Here's how the part is built. I have some questions about the finished solid (model axes, mm). Round coordinates to 2 decimals unless told otherwise and drop trailing zeros. Order: outer loops, then holes, each group sorted by start corner. A loop starts at its lowest first (then second) coordinate and runs counter-clockwise, first axis right, second up. Notation, with made-up numbers: (-18, -26) -> (15, -26) arc R7 cw to (15, -22) -> close; hole circle Ø8 at (87, 76). An arc over 180 degrees is marked (long way). Use a Markdown table: item, result. Add a question column.
(1) I'm going to push flat-ended pins straight in: P1, Ø3.5, axis at x = -5, z = 8, coming from the +Y side; P2, Ø10, axis at y = 72, z = 5, coming from the +X side; P3, Ø5, axis at x = -40.5, y = -55.5, coming from the +Z side; P4, Ø4.5, axis at y = -86.36, z = 11.11, coming from the -X side. Where does each tip first touch, or does it pass through?
(2) I want a section at B-B, the plane x = 0. Please give me the cut outline in (y, z).
(3) I want a section at A-A, the plane y = 86.36. Give the number of separate pieces and of enclosed holes in the cut face, then the cut area to 3 significant figures.
(4) I want a section at D-D, the plane x = 69. Please give me the cut outline in (y, z).
(5) If I drill on probe 1 along Z at (x, y) = (5.1, 86.36); probe 2 along Z at (x, y) = (-1, -31.5); probe 3 along Z at (x, y) = (4, -86), over which ranges is the centre line in solid material (lowest first)?
from build123d import *

# Parameters (mm, degrees)
F0_W     = 203.2
F0_H     = 203.2
F1_DEPTH = 4.7625
F2_W     = 17.78
F2_H     = 12.7
F3_DEPTH = 6.35
F4_W     = 6.35
F4_H     = 17.78
F4_W_2   = 3.175
F5_DEPTH = 12.7
F7_D     = 4.7625
F9_DEPTH = 4.7635
F10_R    = 6.35
F12_D    = 2.794


with BuildPart() as f1:
    # F0 (on Top) → F1 (new body)
    with BuildSketch(Plane.XY):
        Rectangle(F0_W, F0_H)
    extrude(amount=F1_DEPTH)

    # F2 (on Right) → F3 (join, symmetric)
    with BuildSketch(Plane.YZ):
        with Locations((-86.36, 11.1125)):
            Rectangle(F2_W, F2_H)
        with Locations((86.36, 11.1125)):
            Rectangle(F2_W, F2_H)
    extrude(amount=F3_DEPTH, both=True)

    # F4 (on face) → F5 (cut, through all)
    with BuildSketch(Plane.XY.offset(17.4625)):
        with Locations((0, -86.36)):
            Rectangle(F4_W, F4_H)
        with Locations((-1.5875, 86.36)):
            Rectangle(F4_W_2, F4_H)
        with Locations((1.5875, 86.36)):
            Rectangle(F4_W_2, F4_H)
    extrude(amount=-F5_DEPTH, mode=Mode.SUBTRACT)

    # F7 (through all)
    with Locations(Plane.YZ.offset(6.35)):
        with Locations((-86.36, 11.1125), (86.36, 11.1125)):
            Hole(F7_D / 2)

    # F8 (on face) → F9 (cut, through all)
    with BuildSketch(Plane.XY.offset(4.7625)):
        with BuildLine():
            Line((-101.6, -101.6), (-3.53e-08, -101.6))
            ThreePointArc((-3.53e-08, -101.6), (-71.842048981, -71.8420489561), (-101.6, 0))
            Line((-101.6, 0), (-101.6, -101.6))
        make_face()
        with BuildLine():
            ThreePointArc((-101.6, 0), (-71.8420489199, 71.8420490172), (1.376e-07, 101.6))
            Line((1.376e-07, 101.6), (-101.6, 101.6))
            Line((-101.6, 101.6), (-101.6, 0))
        make_face()
        with BuildLine():
            ThreePointArc((1.376e-07, 101.6), (71.8420490172, 71.8420489199), (101.6, 0))
            Line((101.6, 0), (101.6, 101.6))
            Line((101.6, 101.6), (1.376e-07, 101.6))
        make_face()
        with BuildLine():
            Line((101.6, -101.6), (101.6, 0))
            ThreePointArc((101.6, 0), (71.8420489561, -71.842048981), (-3.53e-08, -101.6))
            Line((-3.53e-08, -101.6), (101.6, -101.6))
        make_face()
    extrude(amount=-F9_DEPTH, mode=Mode.SUBTRACT)

    # F10
    f10_edges = [f1.edges().sort_by_distance(p)[0] for p in [
        (-4.7625, -95.25, 17.4625),
        (-4.7625, -77.47, 17.4625),
        (-4.7625, 77.47, 17.4625),
        (-4.7625, 95.25, 17.4625),
        (4.7625, 95.25, 17.4625),
        (4.7625, 77.47, 17.4625),
        (4.7625, -95.25, 17.4625),
        (4.7625, -77.47, 17.4625),
    ]]
    fillet(f10_edges, radius=F10_R)

    # F12 (through all)
    with Locations(Plane.XY.offset(4.7625)):
        with Locations((-88.9, 0), (88.9, 0), (-96.52, 0), (96.52, 0)):
            Hole(F12_D / 2)


solid = f1.part
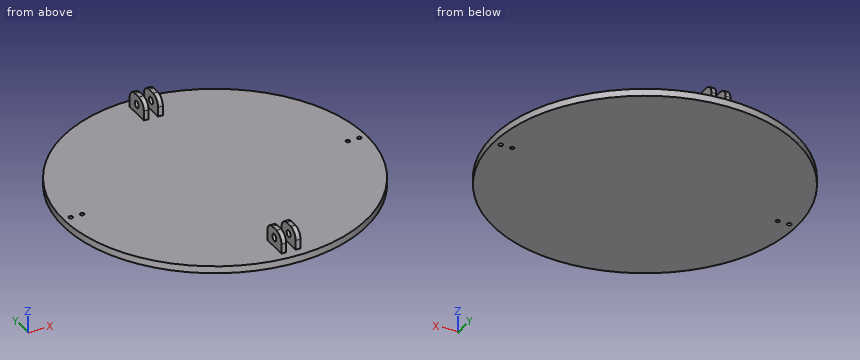
Taken from the geometry:
| question | item | result |
|---|---|---|
| 1 | P1 | stops at y = 95.25 |
| 1 | P2 | stops at x = 76.37 |
| 1 | P3 | stops at z = 4.76 |
| 1 | P4 | passes through |
| 2 | outline | (-101.6, 0) -> (101.6, 0) -> (101.6, 4.76) -> (-101.6, 4.76) -> close |
| 3 | separate pieces | 3 |
| 3 | enclosed holes | 0 |
| 3 | area | 560 mm2 |
| 4 | outline | (-74.58, 0) -> (74.58, 0) -> (74.58, 4.76) -> (-74.58, 4.76) -> close |
| 5 | probe 1 | z = 0 to 8.73, 13.49 to 17.46 |
| 5 | probe 2 | z = 0 to 4.76 |
| 5 | probe 3 | z = 0 to 8.76, 13.47 to 17.46 |
